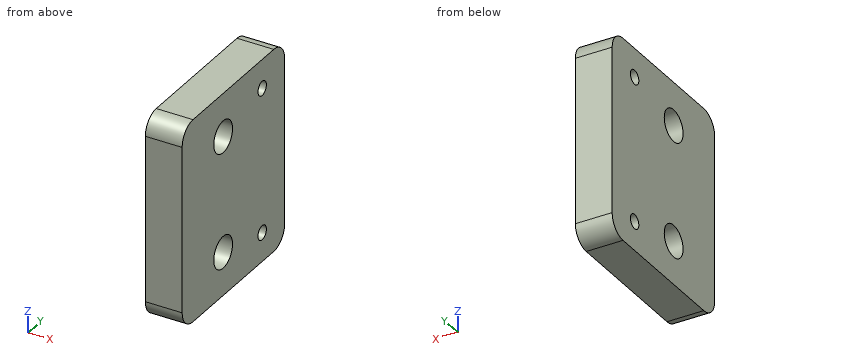
Autodesk Inventor part; units mm, degrees
ref_plane "YZ Plane" through (0, 0, 0) normal (1, 0, 0) x (0, 1, 0)
ref_plane "XZ Plane" through (0, 0, 0) normal (0, 1, 0) x (-1, 0, 0)
ref_plane "XY Plane" through (0, 0, 0) normal (0, 0, 1) x (1, 0, 0)
sketch "Sketch1" plane through (0, 0, 0) normal (1, 0, 0) x (0, 1, 0)
  line L0 (-12, 17.5) -> (18, 17.5)
  line L1 (18, 17.5) -> (18, -17.5)
  line L2 (18, -17.5) -> (-12, -17.5)
  line L3 (-12, -17.5) -> (-12, 17.5)
  point P0 (0, 0)
  dimension "d0" = 35
  dimension "d1" = 30
  dimension "d3" = 17.5
  dimension "d7" = 18
extrude "Extrusion1" add sketch "Sketch1" along normal blind 6.35
fillet "Fillet1" radius 3.175 4 edges at (3.175, -12, -17.5) (3.175, -12, 17.5) (3.175, 18, 17.5) (3.175, 18, -17.5)
sketch "Sketch2" plane through (6.35, 0, 0) normal (1, 0, 0) x (0, 0, -1)
  point P0 (0, 0)
  point P1 (-10, 0)
  point P2 (10, 0)
  dimension "d15" = 20
  dimension "d16" = 10
hole "Hole1" at (6.35, 0, 10) at (6.35, 0, -10) direction (-1, 0, 0) diameter 5.5118 end through all
sketch "Sketch3" plane through (6.35, 0, 0) normal (1, 0, 0) x (0, 0, -1)
  point P0 (0, 0)
  point P1 (-12.5, 11.43)
  point P2 (12.5, 11.43)
  dimension "d17" = 25
  dimension "d18" = 12.5
  dimension "d19" = 11.43
hole "Hole2" at (6.35, 11.43, 12.5) at (6.35, 11.43, -12.5) direction (-1, 0, 0) diameter 2.459 end through all
properties material "ABS, BLACK"
Geometry check sheet. Reference: the model listing, model coordinates, mm. Round coordinates to 2 decimals unless told otherwise and drop trailing zeros. Write each loop counter-clockwise with the first axis right and the second up, starting at its lowest first coordinate (ties: lowest second). Pieces come first, ordered by that corner, then holes.
Item 1: Section check A-A (z = -10). Record the boundary of the cut face in (x, y), plus the area to 4 significant figures.
Determined:
outline: (0, -12) - (6.35, -12) - (6.35, -2.76) - (0, -2.76) - close; (0, 2.76) - (6.35, 2.76) - (6.35, 18) - (0, 18) - close
area: 155.5 mm2
Item 2: Section check C-C (x = 2.25). Give the number of separate pieces and of enclosed holes in the cut face, plus the area to 3 significant figures.
Determined:
separate pieces: 1
enclosed holes: 4
area: 984 mm2
Item 3: Material ranges on line 1 along Z through (x, y) = (3, 11.43); line 2 along Z through (x, y) = (3.5, 0); line 3 along Y through (x, z) = (4.5, 10), recorded low to high.
Determined:
line 1: z = -17.5 to -13.73, -11.27 to 11.27, 13.73 to 17.5
line 2: z = -17.5 to -12.76, -7.24 to 7.24, 12.76 to 17.5
line 3: y = -12 to -2.76, 2.76 to 18
Item 4: Section check B-B (y = 11.43). Record the boundary of the cut face in (x, z).
Determined:
outline: (0, -17.5) - (6.35, -17.5) - (6.35, -13.73) - (0, -13.73) - close; (0, -11.27) - (6.35, -11.27) - (6.35, 11.27) - (0, 11.27) - close; (0, 13.73) - (6.35, 13.73) - (6.35, 17.5) - (0, 17.5) - close
Item 5: Section check D-D (y = 0). Record the boundary of the cut face in (x, z), plus the area to 3 significant figures.
Determined:
outline: (0, -17.5) - (6.35, -17.5) - (6.35, -12.76) - (0, -12.76) - close; (0, -7.24) - (6.35, -7.24) - (6.35, 7.24) - (0, 7.24) - close; (0, 12.76) - (6.35, 12.76) - (6.35, 17.5) - (0, 17.5) - close
area: 152 mm2
